```python
from build123d import *

# Parameters (mm, degrees)
F0_R     = 11
F1_DEPTH = 7


with BuildPart() as f1:
    # F0 (on Top) → F1 (new body)
    with BuildSketch(Plane.XY):
        with BuildLine():
            ThreePointArc((-24.363253, -11.132389), (-20.055418, -6.291022), (-18.5, 0))
            ThreePointArc((-18.5, 0), (-19.935078, 6.057035), (-23.93521, 10.826318))
            ThreePointArc((-23.93521, 10.826318), (-45.497436, 0.263106), (-24.363253, -11.132389))
        make_face()
        with Locations((-32, 0)):
            Circle(F0_R, mode=Mode.SUBTRACT)
        with BuildLine():
            ThreePointArc((-23.93521, 10.826318), (-19.935078, 6.057035), (-18.5, 0))
            ThreePointArc((-18.5, 0), (-20.055418, -6.291022), (-24.363253, -11.132389))
            ThreePointArc((-24.363253, -11.132389), (-16.075993, -9.03197), (-7.766423, -11.042313))
            ThreePointArc((-7.766423, -11.042313), (-13.498744, -0.184171), (-8.06479, 10.826318))
            ThreePointArc((-8.06479, 10.826318), (-16, 8.957347), (-23.93521, 10.826318))
        make_face()
        with BuildLine():
            ThreePointArc((8.06479, 10.826318), (0, 13.5), (-8.06479, 10.826318))
            ThreePointArc((-8.06479, 10.826318), (-13.498744, -0.184171), (-7.766423, -11.042313))
            ThreePointArc((-7.766423, -11.042313), (0.073268, -13.499801), (7.885822, -10.957363))
            ThreePointArc((7.885822, -10.957363), (12.014753, -6.155948), (13.5, 0))
            ThreePointArc((13.5, 0), (12.064922, 6.057035), (8.06479, 10.826318))
        make_face()
        Circle(F0_R, mode=Mode.SUBTRACT)
        with BuildLine():
            ThreePointArc((23.93521, 10.826318), (16, 8.957347), (8.06479, 10.826318))
            ThreePointArc((8.06479, 10.826318), (12.064922, 6.057035), (13.5, 0))
            ThreePointArc((13.5, 0), (12.014753, -6.155948), (7.885822, -10.957363))
            ThreePointArc((7.885822, -10.957363), (15.929492, -8.984778), (23.994099, -10.869938))
            ThreePointArc((23.994099, -10.869938), (18.50005, -0.036642), (23.93521, 10.826318))
        make_face()
        with BuildLine():
            ThreePointArc((45.5, 0), (38.057035, 12.064922), (23.93521, 10.826318))
            ThreePointArc((23.93521, 10.826318), (18.50005, -0.036642), (23.994099, -10.869938))
            ThreePointArc((23.994099, -10.869938), (38.08976, -12.048437), (45.5, 0))
        make_face()
        with Locations((32, 0)):
            Circle(F0_R, mode=Mode.SUBTRACT)
    extrude(amount=F1_DEPTH)


solid = f1.part
```
Could you check a few things on this model? Use its own coordinates, in mm. Give positions to 0.01 mm unless a question says otherwise; leave off trailing zeros. Loops run counter-clockwise (first coordinate to the right, second up) from the corner with the lowest first, then second, coordinate; pieces in that order, holes last. Notation, with made-up numbers: (-2.5, 51.25) - (38.5, 51.25) arc R5 ccw to (38.5, 56.25) - close; hole circle Ø8 at (83.5, 62.25). An arc over 180 degrees is marked (long way). Use one line per item in the form item = value.
1. I want a section at C-C (z = 4.5). Please give me the cut outline in (x, y).
Response values:
outline = (-24.36, -11.13) arc R17.78 cw to (-7.77, -11.04) arc R13.5 ccw to (7.89, -10.96) arc R17.78 cw to (23.99, -10.87) arc R13.5 ccw to (45.5, 0) arc R13.5 ccw to (23.94, 10.83) arc R17.78 cw to (8.06, 10.83) arc R13.5 ccw to (-8.06, 10.83) arc R17.78 cw to (-23.94, 10.83) arc R13.5 ccw (long way) to start; hole circle Ø22 at (-32, 0); hole circle Ø22 at (0, 0); hole circle Ø22 at (32, 0)
2. Thinking about a two-plate mould opening in X: for faces 1 (the face through (-11, -3, 7)), 2 (the face through (16.115, 8.958, 3.451)), which applies, released by +X, released by -X, zero draft, split by the parting line, or undercut?
Response values:
face_1 = zero draft
face_2 = undercut
3. I'm going to push flat-ended pins straight in: pin 1 Ø1.5 at (x, y) = (1, -9) entering from -Z; pin 2 Ø4 at (y, z) = (8, 6) entering from -X; pin 3 Ø1.5 at (x, z) = (11.5, 1) entering from -Y; pin 4 Ø1 at (x, z) = (-7, 4.5) entering from +Y. Where does each tip first touch, or does it pass through?
Response values:
pin_1 = through
pin_2 = -44.09
pin_3 = -9.79
pin_4 = 11.83
4. I want a section at D-D (x = 38). Please give me the cut outline in (y, z).
Response values:
outline = (-12.09, 0) - (-9.22, 0) - (-9.22, 7) - (-12.09, 7) - close; (9.22, 0) - (12.09, 0) - (12.09, 7) - (9.22, 7) - close
5. I need wall thicknesses on probe 1 along X at (y, z) = (0.75, 4.5); probe 2 along Y at (x, z) = (-32, 4.75); probe 3 along X at (y, z) = (-3.25, 4.5). Which ranges of each line are inside material? Lowest first, please.
Response values:
probe_1 = -45.48 to -42.97, -21.03 to -10.97, 10.97 to 21.03, 42.97 to 45.48
probe_2 = -13.5 to -11, 11 to 13.5
probe_3 = -45.1 to -42.51, -21.49 to -10.51, 10.51 to 21.49, 42.51 to 45.1
6. I want a section at A-A (x = -32). Please give me the cut outline in (y, z), and give its area (3 significant figures).
Response values:
outline = (-13.5, 0) - (-11, 0) - (-11, 7) - (-13.5, 7) - close; (11, 0) - (13.5, 0) - (13.5, 7) - (11, 7) - close
area = 35.0 mm²
7. I want a section at B-B (y = 3.5). Please give me the cut outline in (x, z), and give its area (3 significant figures).
Response values:
outline = (-45.04, 0) - (-42.43, 0) - (-42.43, 7) - (-45.04, 7) - close; (-21.57, 0) - (-10.43, 0) - (-10.43, 7) - (-21.57, 7) - close; (10.43, 0) - (21.57, 0) - (21.57, 7) - (10.43, 7) - close; (42.43, 0) - (45.04, 0) - (45.04, 7) - (42.43, 7) - close
area = 193 mm²
